For this review, use the dimensioned drawing (mm, ordinates from the lowest corner) and the shaded views. A direction names the side the tool comes from. Give positions to 0.01 mm unless a question says otherwise; leave off trailing zeros. Order: outer loops, then holes, each group sorted by start corner. A loop starts at its lowest first (then second) coordinate and runs counter-clockwise, first axis right, second up. Notation, with made-up numbers: (-38, 37) - (-5, 37) arc R24 cw to (-5, 63) - close; hole circle Ø7 at (67.25, 89). An arc over 180 degrees is marked (long way). Use a Markdown table: item, result. Add a question column.
1) Machinability: for the marked faces 1, 2 and 3, which of the approach directions +Z, -Z, +X, -X, +Y, -Y give a long, thin tool a straight path to every point of the face, cutting with its end or side? Answer none if there is none.
2) Clearance check with flat-ended pins moving along their axes: P1, Ø1.5, axis at x = 9, y = 32.5, coming from the +Z side; P2, Ø1.5, axis at x = 4.5, y = 21.5, coming from the -Z side; P3, Ø2, axis at x = 2.5, y = 35.5, coming from the +Z side. State where each tip first meets the part, or that it passes through.
3) We need section B-B on x = 6. Write out the cut boundary in (y, z), then the cut area to 3 significant figures.
4) We need section D-D on z = 10.75. Write out the cut boundary in (x, y), then the cut area to 3 significant figures.
5) Wall thickness on L1, parallel to Y at x = 6, z = 10.5; L2, parallel to Z at x = 8, y = 48: over which ranges is each line inside the solid? List them lowest first.
6) We need section C-C on y = 19.5. Write out the cut boundary in (x, z).
7) We need section A-A on z = 6. Write out the cut boundary in (x, y), then the cut area to 3 significant figures.
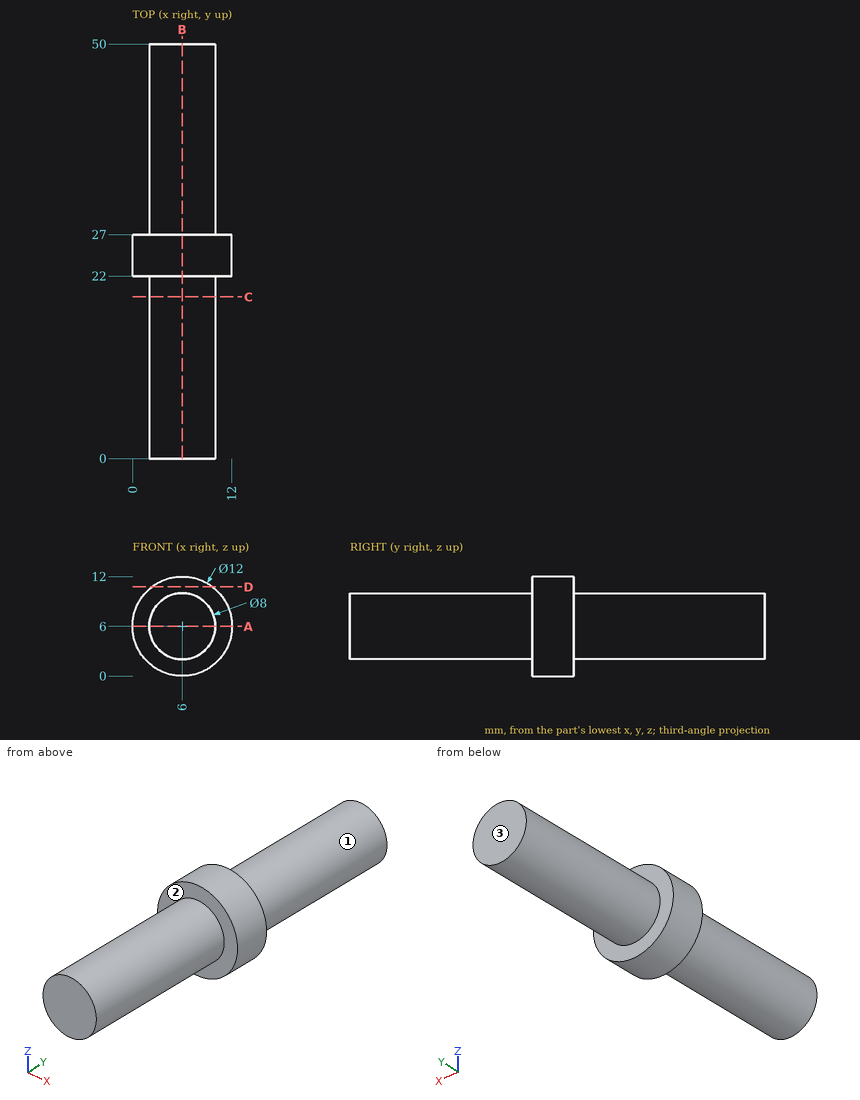
Checked values:
| question | item | result |
|---|---|---|
| 1 | face 1 | +Y |
| 1 | face 2 | -Y |
| 1 | face 3 | +Z, -Z, +X, -X, +Y |
| 2 | P1 | z = 9.31 |
| 2 | P2 | z = 0.07 |
| 2 | P3 | z = 9.12 |
| 3 | outline | (0, 2) - (22, 2) - (22, 0) - (27, 0) - (27, 2) - (50, 2) - (50, 10) - (27, 10) - (27, 12) - (22, 12) - (22, 10) - (0, 10) - close |
| 3 | area | 420 mm² |
| 4 | outline | (2.33, 22) - (9.67, 22) - (9.67, 27) - (2.33, 27) - close |
| 4 | area | 36.7 mm² |
| 5 | L1 | 22 to 27 |
| 5 | L2 | 2.54 to 9.46 |
| 6 | outline | circle Ø8 at (6, 6) |
| 7 | outline | (0, 22) - (2, 22) - (2, 0) - (10, 0) - (10, 22) - (12, 22) - (12, 27) - (10, 27) - (10, 50) - (2, 50) - (2, 27) - (0, 27) - close |
| 7 | area | 420 mm² |
